Could you check a few things on this drawing? It's one solid part, dimensions in mm from its lowest x, y, z. Round coordinates to 2 decimals unless told otherwise and drop trailing zeros. Loops run counter-clockwise (first coordinate to the right, second up) from the corner with the lowest first, then second, coordinate; pieces in that order, holes last. Notation, with made-up numbers: M -6,88.5 L 40,88.5 A9 cw 40,98.5 Z; hole C -2.75,-7 d2. An arc over 180 degrees is marked long. Use a Markdown table: item, result. Add a question column.
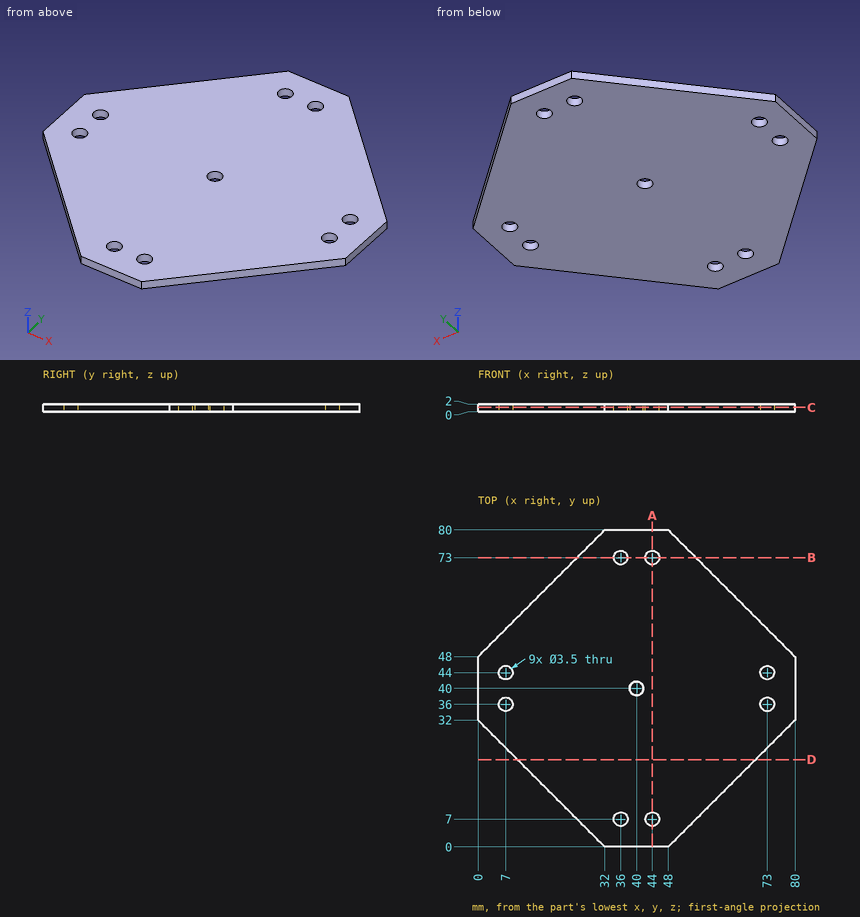
(1) I'm going to push flat-ended pins straight in: pin 1 (3 mm diameter, centred on x = 7, y = 44, fed in from -Z) (1 decimal); pin 2 (1 mm diameter, centred on x = 68.5, z = 1, fed in from +Y). Where does each tip first touch, or does it pass through?
(2) Suppose I cut it at C-C on z = 1.15. Count the separate pieces of the cut face and the enclosed holes in it, and give its area (3 significant figures).
(3) Suppose I cut it at B-B on y = 73. List the corners of the cut face in (x, z) for me.
(4) Suppose I cut it at D-D on y = 22. List the corners of the cut face in (x, z) for me.
(5) If I drill on probe 1 along X at (y, z) = (36, 1.2); probe 2 along Y at (x, z) = (73, 1.3), over which ranges is the centre line in solid material (lowest first)? Write a range as [from, to].
(6) Suppose I cut it at A-A on x = 44. List the corners of the cut face in (y, z) for me.
Results below:
| question | item | result |
|---|---|---|
| 1 | pin 1 | passes through |
| 1 | pin 2 | stops at y = 60 |
| 2 | separate pieces | 1 |
| 2 | enclosed holes | 9 |
| 2 | area | 4,270 mm² |
| 3 | outline | M 25,0 L 34.25,0 L 34.25,2 L 25,2 Z; M 37.75,0 L 42.25,0 L 42.25,2 L 37.75,2 Z; M 45.75,0 L 55,0 L 55,2 L 45.75,2 Z |
| 4 | outline | M 10,0 L 70,0 L 70,2 L 10,2 Z |
| 5 | probe 1 | x = [0, 5.25], [8.75, 71.25], [74.75, 80] |
| 5 | probe 2 | y = [25, 34.25], [37.75, 42.25], [45.75, 55] |
| 6 | outline | M 0,0 L 5.25,0 L 5.25,2 L 0,2 Z; M 8.75,0 L 71.25,0 L 71.25,2 L 8.75,2 Z; M 74.75,0 L 80,0 L 80,2 L 74.75,2 Z |
